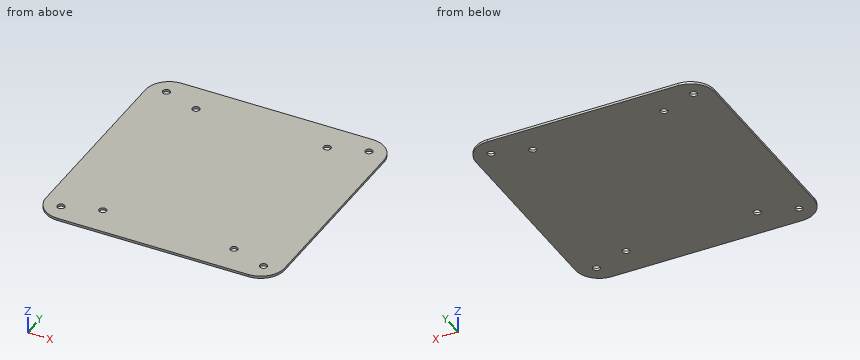
```python
from build123d import *

# Parameters (mm, degrees)
SKETCH_1_R      = 1.55
EXTRUDE_1_DEPTH = 1


with BuildPart() as part:
    # 草图1 → 凸台-拉伸1 (new body)
    with BuildSketch(Plane.XY):
        with BuildLine():
            Line((-40, -50), (40, -50))
            ThreePointArc((40, -50), (47.071067812, -47.071067812), (50, -40))
            Line((50, -40), (50, 40))
            ThreePointArc((50, 40), (47.071067812, 47.071067812), (40, 50))
            Line((40, 50), (-40, 50))
            ThreePointArc((-40, 50), (-47.071067812, 47.071067812), (-50, 40))
            Line((-50, 40), (-50, -40))
            ThreePointArc((-50, -40), (-47.071067812, -47.071067812), (-40, -50))
        make_face()
        with Locations((-27.5, 37.5)):
            Circle(SKETCH_1_R, mode=Mode.SUBTRACT)
        with Locations((27.5, 37.5)):
            Circle(SKETCH_1_R, mode=Mode.SUBTRACT)
        with Locations((27.5, -37.5)):
            Circle(SKETCH_1_R, mode=Mode.SUBTRACT)
        with Locations((-27.5, -37.5)):
            Circle(SKETCH_1_R, mode=Mode.SUBTRACT)
        with Locations((-42.426406871, 42.426406871)):
            Circle(SKETCH_1_R, mode=Mode.SUBTRACT)
        with Locations(Location((42.426406871, 42.426406871, 0), (0, 0, 180))):
            Circle(SKETCH_1_R, mode=Mode.SUBTRACT)
        with Locations((42.426406871, -42.426406871)):
            Circle(SKETCH_1_R, mode=Mode.SUBTRACT)
        with Locations(Location((-42.426406871, -42.426406871, 0), (0, 0, 180))):
            Circle(SKETCH_1_R, mode=Mode.SUBTRACT)
    extrude(amount=EXTRUDE_1_DEPTH)


solid = part.part
```
Model file for the job. Use its own axes, mm. Coordinates: 2 decimals unless noted, no trailing zeros. Order: outer loops, then holes, each group sorted by start corner. A loop starts at its lowest first (then second) coordinate and runs counter-clockwise, first axis right, second up. Notation, with made-up numbers: (-4.75, 84) -> (19.25, 84) arc R34 cw to (19.25, 122) -> close; hole circle Ø9 at (60, -10). An arc over 180 degrees is marked (long way). Answer as a JSON object with one key per item and string values. Group by question number.
1) Cut at B-B, the plane y = -37.5. Write the cut outline in (x, z).
2) Drill centre lines: L1, parallel to Y at x = -42, z = 0.75; L2, parallel to X at y = -42.5, z = 0.25. Where is each one in solid material? Low to high.
3) Cut at A-A, the plane x = 27.5. Write the cut outline in (y, z).
4) Flat gauge pin, fed straight in: pin 1 (2.5 mm diameter, centred on x = -42.43, y = 42.43, fed in from -Z). Where does the tip first touch, or does it go through?
Check values:
{
 "1": {"outline": "(-50, 0) -> (-29.05, 0) -> (-29.05, 1) -> (-50, 1) -> close; (-25.95, 0) -> (25.95, 0) -> (25.95, 1) -> (-25.95, 1) -> close; (29.05, 0) -> (50, 0) -> (50, 1) -> (29.05, 1) -> close"},
 "2": {"L1": "y = -49.8 to -43.92, -40.94 to 40.94, 43.92 to 49.8", "L2": "x = -49.68 to -43.97, -40.88 to 40.88, 43.97 to 49.68"},
 "3": {"outline": "(-50, 0) -> (-39.05, 0) -> (-39.05, 1) -> (-50, 1) -> close; (-35.95, 0) -> (35.95, 0) -> (35.95, 1) -> (-35.95, 1) -> close; (39.05, 0) -> (50, 0) -> (50, 1) -> (39.05, 1) -> close"},
 "4": {"pin 1": "passes through"}
}
